The listing builds one solid part. Answer for the finished solid, in the listing's coordinates (mm). A direction names the side the tool comes from. Coordinates: 2 decimals unless noted, no trailing zeros. Write each loop counter-clockwise with the first axis right and the second up, starting at its lowest first coordinate (ties: lowest second). Pieces come first, ordered by that corner, then holes.
(1) For a pull along Z with two mould halves and no side action, classify faces 1 (the flat face through (25.8, 10, -4)), 2 (the cylindrical face through (13.786, -8.244, -6.414)), 3 (the flat face through (13, 7, -7.2)) as +Z half, -Z half, draft (parallel to the pull), parting line (faces both ways), or undercut.
(2) Which of the six approach directions +Z, -Z, +X, -X, +Y, -Y give full straight-line access (tool end or side, diameter ignored) to faces 4 (the flat face through (1.65, 12, -4)), 5 (the cylindrical face through (4.582, -7.678, -0.451))?
(3) The part is cut by section A-A on y = 10.2. Determine the outline of the cut face in (x, z), plus the area to 3 significant figures.
(4) The part is cut by section C-C on z = -3.6. Determine the outline of the cut face in (x, y), plus the area to 3 significant figures.
(5) The part is cut by section D-D on x = 12.9. Determine the outline of the cut face in (y, z).
(6) The part is cut by section B-B on y = 3. Determine the outline of the cut face in (x, z).
(7) Given P1, Ø10, axis at x = 19.5, y = 13, coming from the +Z side; P2, Ø4, axis at x = 6, y = -0.5, coming from the -Z side; P3, Ø1.8, axis at x = 11.5, z = -3, coming from the -Y side; P4, Ø1.8, axis at x = 12.95, y = 10.2, coming from the -Z side, each flat-ended and moving along its own axis, determine where each tip first touches the part or whether it passes through.
(8) Straight lines are drawn through the part: line 1 (Z direction, x = 17.5, y = 18); line 2 (X direction, y = 16, z = -3.25). For each, find the intervals that lie inside material, in ascending order.
from build123d import *

# Parameters (mm, degrees)
SKETCH2_W               = 25.8
SKETCH2_H               = 7.2
BOSS_EXTRUDE1_DEPTH     = 20.5
SKETCH3_W               = 22.5
SKETCH3_H               = 3.3
CUT_EXTRUDE1_DEPTH      = 18
CUT_EXTRUDE2_DEPTH      = 34.730253483
CUT_EXTRUDE2_DEPTH_BACK = 34.730253483
SKETCH4_R               = 1
SKETCH9_R               = 4.95
BOSS_EXTRUDE6_DEPTH     = 14.9
BOSS_EXTRUDE7_DEPTH     = 7.2
SKETCH12_R              = 2.95
CUT_EXTRUDE5_DEPTH      = 13.5
FILLET2_R               = 1.5
FILLET3_R               = 1.8


with BuildPart() as part:
    # Sketch2 → Boss-Extrude1 (new body)
    with BuildSketch(Plane(origin=(0, 0, 0), x_dir=(1, 0, 0), z_dir=(0, 1, 0))):
        with Locations((12.9, 3.6)):
            Rectangle(SKETCH2_W, SKETCH2_H)
    extrude(amount=BOSS_EXTRUDE1_DEPTH)

    # Sketch3 → Cut-Extrude1 (cut)
    with BuildSketch(Plane(origin=(0, 20.5, 0), x_dir=(1, 0, 0), z_dir=(0, 1, 0))):
        with Locations((12.9, 3.6)):
            Rectangle(SKETCH3_W, SKETCH3_H)
    extrude(amount=-CUT_EXTRUDE1_DEPTH, mode=Mode.SUBTRACT)

    # Sketch4 → Cut-Extrude2 (cut, two sides: drawn at the far end of the back side and taken through both)
    with BuildSketch(Plane(origin=(0, 0, -7.2), x_dir=(-1, 0, 0), z_dir=(0, 0, -1)).offset(-CUT_EXTRUDE2_DEPTH_BACK)):
        with Locations((-12.953971153, 10.2)):
            Circle(SKETCH4_R)
    extrude(amount=CUT_EXTRUDE2_DEPTH + CUT_EXTRUDE2_DEPTH_BACK, mode=Mode.SUBTRACT)

    # Sketch9 → Boss-Extrude6 (add)
    with BuildSketch(Plane(origin=(0, 0, 0), x_dir=(-1, 0, 0), z_dir=(0, -1, 0))):
        with Locations(Location((-12.9, 3.6, 0), (0, 0, 226.658241773))):
            Circle(SKETCH9_R)
    extrude(amount=BOSS_EXTRUDE6_DEPTH)

    # Sketch11 → Boss-Extrude7 (add)
    with BuildSketch(Plane(origin=(0, 0, -7.2), x_dir=(-1, 0, 0), z_dir=(0, 0, -1))):
        Polygon((-9.502574504, 0), (-12.9, 0), (-12.9, -14.9), (-7.95, -14.9), (0, 0), align=None)
        Polygon((-12.9, -14.9), (-12.9, 0), (-16.297425496, 0), (-25.8, 0), (-17.85, -14.9), align=None)
    extrude(amount=-BOSS_EXTRUDE7_DEPTH)

    # Sketch12 → Cut-Extrude5 (cut)
    with BuildSketch(Plane(origin=(0, -14.9, 0), x_dir=(-1, 0, 0), z_dir=(0, -1, 0))):
        with Locations(Location((-12.9, 3.6, 0), (0, 0, 90))):
            Circle(SKETCH12_R)
    extrude(amount=-CUT_EXTRUDE5_DEPTH, mode=Mode.SUBTRACT)

    # Fillet2
    # the kernel refuses this fillet: 1.5 mm, written as the material it takes off along each edge
    with BuildSketch(Plane(origin=(0, -3.75, -7.2), x_dir=(0, 0, 1), z_dir=(0, 1, 0)), Plane(origin=(0, -3.75, 0), x_dir=(1, 0, 0), z_dir=(0, 1, 0))) as fillet2_piece_1:
        with BuildLine():
            CenterArc((FILLET2_R, FILLET2_R), FILLET2_R, 180, 90)
            Line((0, FILLET2_R), (0, 0))
            Line((0, 0), (FILLET2_R, 0))
        make_face()
    extrude(amount=28, mode=Mode.SUBTRACT)
    with BuildSketch(Plane(origin=(9.715282105, -18.208516146, -7.2), x_dir=(0, 0, 1), z_dir=(-0.47074189463756383, 0.8822709723395851, 0))) as fillet2_piece_2_section:
        with BuildLine():
            CenterArc((FILLET2_R, FILLET2_R), FILLET2_R, 180, 90)
            Line((0, FILLET2_R), (0, 0))
            Line((0, 0), (FILLET2_R, 0))
        make_face()
    fillet2_piece_2 = extrude(amount=24.38823555, mode=Mode.PRIVATE)
    fillet2_piece_2 = fillet2_piece_2 - Plane(origin=(12.9, -7.082671963, -3.6), x_dir=(0.686348585021791, 0, 0.727272727275391), z_dir=(0, 1, 0)) * Cylinder(4.95, 55, mode=Mode.PRIVATE)
    add(fillet2_piece_2, mode=Mode.SUBTRACT)
    with BuildSketch(Plane(origin=(9.715282105, -18.208516146, 0), x_dir=(0.8822709723395851, 0.4707418946375639, 0), z_dir=(-0.47074189463756383, 0.8822709723395851, 0))) as fillet2_piece_3_section:
        with BuildLine():
            CenterArc((FILLET2_R, FILLET2_R), FILLET2_R, 180, 90)
            Line((0, FILLET2_R), (0, 0))
            Line((0, 0), (FILLET2_R, 0))
        make_face()
    fillet2_piece_3 = extrude(amount=24.38823555, mode=Mode.PRIVATE)
    fillet2_piece_3 = fillet2_piece_3 - Plane(origin=(12.9, -7.08267196, -3.6), x_dir=(0.686348585021791, 0, 0.727272727275391), z_dir=(0, 1, 0)) * Cylinder(4.95, 55, mode=Mode.PRIVATE)
    add(fillet2_piece_3, mode=Mode.SUBTRACT)
    with BuildSketch(Plane(origin=(27.565282105, 3.308516146, -7.2), x_dir=(0, 0, 1), z_dir=(-0.4707418946375641, -0.882270972339585, 0))) as fillet2_piece_4_section:
        with BuildLine():
            CenterArc((FILLET2_R, FILLET2_R), FILLET2_R, 180, 90)
            Line((0, FILLET2_R), (0, 0))
            Line((0, 0), (FILLET2_R, 0))
        make_face()
    fillet2_piece_4 = extrude(amount=24.38823555, mode=Mode.PRIVATE)
    fillet2_piece_4 = fillet2_piece_4 - Plane(origin=(12.9, -7.082671987, -3.6), x_dir=(0.686348585021791, 0, 0.727272727275391), z_dir=(0, 1, 0)) * Cylinder(4.95, 55, mode=Mode.PRIVATE)
    add(fillet2_piece_4, mode=Mode.SUBTRACT)
    with BuildSketch(Plane(origin=(27.565282105, 3.308516146, 0), x_dir=(-0.8822709723395848, 0.47074189463756405, 0), z_dir=(-0.4707418946375641, -0.882270972339585, 0))) as fillet2_piece_5_section:
        with BuildLine():
            CenterArc((FILLET2_R, FILLET2_R), FILLET2_R, 180, 90)
            Line((0, FILLET2_R), (0, 0))
            Line((0, 0), (FILLET2_R, 0))
        make_face()
    fillet2_piece_5 = extrude(amount=24.38823555, mode=Mode.PRIVATE)
    fillet2_piece_5 = fillet2_piece_5 - Plane(origin=(12.9, -7.082671971, -3.6), x_dir=(0.686348585021791, 0, 0.727272727275391), z_dir=(0, 1, 0)) * Cylinder(4.95, 55, mode=Mode.PRIVATE)
    add(fillet2_piece_5, mode=Mode.SUBTRACT)
    with BuildSketch(Plane(origin=(25.8, -3.75, 0), x_dir=(-1, 0, 0), z_dir=(0, 1, 0)), Plane(origin=(25.8, -3.75, -7.2), x_dir=(0, 0, 1), z_dir=(0, 1, 0))) as fillet2_piece_6:
        with BuildLine():
            CenterArc((FILLET2_R, -FILLET2_R), FILLET2_R, 90, 90)
            Line((0, -FILLET2_R), (0, 0))
            Line((0, 0), (FILLET2_R, 0))
        make_face()
    extrude(amount=28, mode=Mode.SUBTRACT)

    # Fillet3
    # the kernel refuses this fillet: 1.8 mm, written as the material it takes off along each edge
    with BuildSketch(Plane(origin=(12.9, 0, -3.6), x_dir=(0.9954823771301547, 0, -0.09494649452874186), z_dir=(-0.09494649452874186, 0, -0.9954823771301547))) as fillet3_piece_1_section:
        with BuildLine():
            CenterArc((4.95 - FILLET3_R, FILLET3_R), FILLET3_R, 270, 90)
            Line((4.95 - FILLET3_R, 0), (4.95, 0))
            Line((4.95, 0), (4.95, FILLET3_R))
        make_face()
    fillet3_piece_1 = revolve(axis=Axis((12.9, 0, -3.6), (0, -1, 0)), revolution_arc=190.896480509, mode=Mode.PRIVATE)
    fillet3_piece_1 = split(fillet3_piece_1, bisect_by=Plane(origin=(12.9, -0.687334204, 0), z_dir=(0, 0, 1)), keep=Keep.TOP, mode=Mode.PRIVATE)
    add(fillet3_piece_1, mode=Mode.SUBTRACT)
    with BuildSketch(Plane(origin=(12.9, 0, -3.6), x_dir=(-0.9954823771297855, 0, 0.09494649453261288), z_dir=(0.09494649453261288, 0, 0.9954823771297855))) as fillet3_piece_2_section:
        with BuildLine():
            CenterArc((4.95 - FILLET3_R, FILLET3_R), FILLET3_R, 270, 90)
            Line((4.95 - FILLET3_R, 0), (4.95, 0))
            Line((4.95, 0), (4.95, FILLET3_R))
        make_face()
    fillet3_piece_2 = revolve(axis=Axis((12.9, 0, -3.6), (0, -1, 0)), revolution_arc=190.89648051, mode=Mode.PRIVATE)
    fillet3_piece_2 = split(fillet3_piece_2, bisect_by=Plane(origin=(12.9, -0.687334204, -7.2), z_dir=(0, 0, -1)), keep=Keep.TOP, mode=Mode.PRIVATE)
    add(fillet3_piece_2, mode=Mode.SUBTRACT)


solid = part.part
Model answer:
1. face 1: draft
1. face 2: undercut
1. face 3: -Z half
2. face 4: +Y
2. face 5: +Z, -X, -Y
3. outline: (0, -5.7) arc R1.5 ccw to (1.5, -7.2) - (11.95, -7.2) - (11.95, -5.25) - (1.65, -5.25) - (1.65, -1.95) - (11.95, -1.95) - (11.95, 0) - (1.5, 0) arc R1.5 ccw to (0, -1.5) - close; (13.95, -7.2) - (24.3, -7.2) arc R1.5 ccw to (25.8, -5.7) - (25.8, -1.5) arc R1.5 ccw to (24.3, 0) - (13.95, 0) - (13.95, -1.95) - (24.15, -1.95) - (24.15, -5.25) - (13.95, -5.25) - close
3. area: 102 mm2
4. outline: (0, 0) - (7.95, -14.9) - (9.95, -14.9) - (9.95, -1.4) - (15.85, -1.4) - (15.85, -14.9) - (17.85, -14.9) - (25.8, 0) - (25.8, 20.5) - (24.15, 20.5) - (24.15, 2.5) - (1.65, 2.5) - (1.65, 20.5) - (0, 20.5) - close
4. area: 310 mm2
5. outline: (-14.9, -8.55) - (-1.8, -8.55) arc R1.8 ccw to (-0.06, -7.2) - (9.2, -7.2) - (9.2, -5.25) - (2.5, -5.25) - (2.5, -1.95) - (9.2, -1.95) - (9.2, 0) - (-0.06, 0) arc R1.8 ccw to (-1.8, 1.35) - (-14.9, 1.35) - (-14.9, -0.65) - (-1.4, -0.65) - (-1.4, -6.55) - (-14.9, -6.55) - close; (11.2, -7.2) - (20.5, -7.2) - (20.5, -5.25) - (11.2, -5.25) - close; (11.2, -1.95) - (20.5, -1.95) - (20.5, 0) - (11.2, 0) - close
6. outline: (0, -5.7) arc R1.5 ccw to (1.5, -7.2) - (24.3, -7.2) arc R1.5 ccw to (25.8, -5.7) - (25.8, -1.5) arc R1.5 ccw to (24.3, 0) - (1.5, 0) arc R1.5 ccw to (0, -1.5) - close; hole (1.65, -5.25) - (24.15, -5.25) - (24.15, -1.95) - (1.65, -1.95) - close
7. P1: stops at z = 0
7. P2: stops at z = -7.2
7. P3: stops at y = -1.4
7. P4: passes through
8. line 1: z = -7.2 to -5.25, -1.95 to 0
8. line 2: x = 0 to 1.65, 24.15 to 25.8
